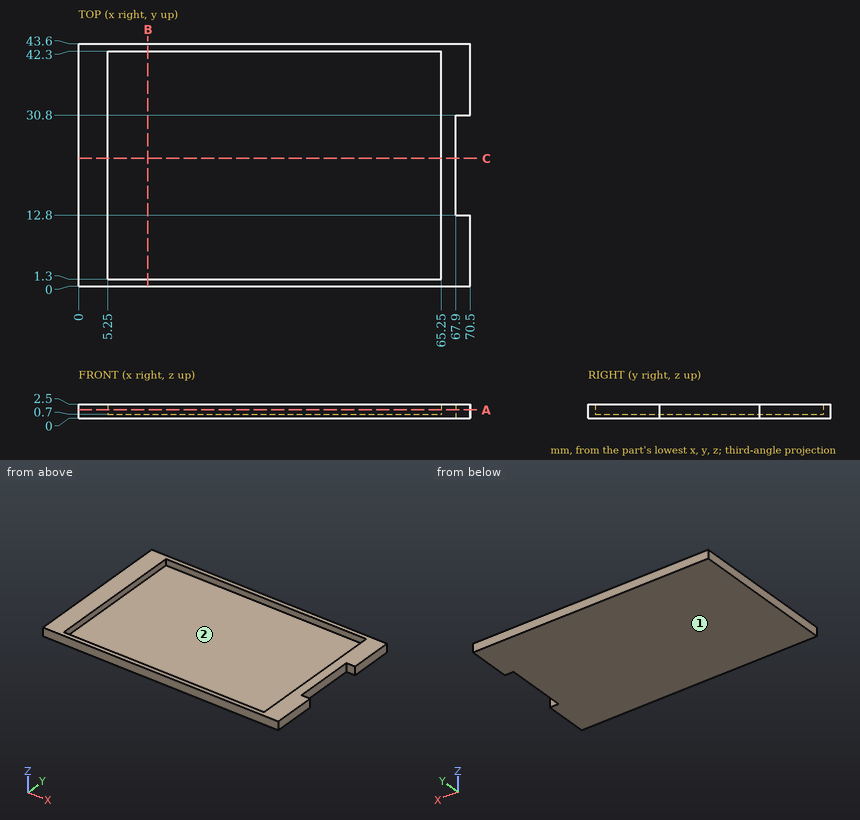
Answer from the drawing. Dimensions are ordinates in mm from the lowest x, y and z of the part. Give positions to 0.01 mm unless a question says otherwise; leave off trailing zeros. Order: outer loops, then holes, each group sorted by start corner. A loop starts at its lowest first (then second) coordinate and runs counter-clockwise, first axis right, second up. Notation, with made-up numbers: (51.25, 81.25) -> (77.25, 81.25) arc R5 cw to (77.25, 89.25) -> close; hole circle Ø7 at (46.5, 62.5). An arc over 180 degrees is marked (long way). One line per item, written item: value. Start each with the question number.
(1) The part is cut by section B-B (x = 12.5). Determine the outline of the cut face in (y, z), and give its area (3 significant figures).
(2) Straight lines are drawn through the part: L1, parallel to Y at x = 8, z = 1.95; L2, parallel to X at y = 32, z = 1.9; L3, parallel to X at y = 23, z = 0.75. For each, find the intervals that lie inside material, in ascending order.
(3) The part is cut by section A-A (z = 1.5). Determine the outline of the cut face in (x, y), and give its area (3 significant figures).
(4) The part is cut by section C-C (y = 23). Determine the outline of the cut face in (x, z), and give its area (4 significant figures).
(5) For a pull along X with two mould halves and no side action, classify the marked faces 1 and 2 as released by +X, released by -X, zero draft, split by the parting line, or undercut.
(6) Flat-ended cylindrical pins translate along their axes: P1, Ø1.4, axis at y = 16, z = 1.5, coming from the +X side; P2, Ø12.5, axis at x = 37.5, y = 24.5, coming from the +Z side. Find the tip coordinate at first contact, or state that the pin passes through.
Taken from the geometry:
1. outline: (0, 0) -> (43.6, 0) -> (43.6, 2.5) -> (42.3, 2.5) -> (42.3, 0.7) -> (1.3, 0.7) -> (1.3, 2.5) -> (0, 2.5) -> close
1. area: 35.2 mm^2
2. L1: 0 to 1.3, 42.3 to 43.6
2. L2: 0 to 5.25, 65.25 to 70.5
2. L3: 0 to 5.25, 65.25 to 67.9
3. outline: (0, 0) -> (70.5, 0) -> (70.5, 12.8) -> (67.9, 12.8) -> (67.9, 30.8) -> (70.5, 30.8) -> (70.5, 43.6) -> (0, 43.6) -> close; hole (5.25, 1.3) -> (65.25, 1.3) -> (65.25, 42.3) -> (5.25, 42.3) -> close
3. area: 567 mm^2
4. outline: (0, 0) -> (67.9, 0) -> (67.9, 2.5) -> (65.25, 2.5) -> (65.25, 0.7) -> (5.25, 0.7) -> (5.25, 2.5) -> (0, 2.5) -> close
4. area: 61.75 mm^2
5. face 1: zero draft
5. face 2: undercut
6. P1: x = 67.9
6. P2: z = 0.7
